Verification items for the finished model (mm, model axes). Give positions to 0.01 mm unless a question says otherwise; leave off trailing zeros. Order: outer loops, then holes, each group sorted by start corner. A loop starts at its lowest first (then second) coordinate and runs counter-clockwise, first axis right, second up. Notation, with made-up numbers: (27.25, 77) -> (70.25, 77) arc R12 ccw to (70.25, 96) -> close; hole circle Ø4 at (28.25, 73.5). An arc over 180 degrees is marked (long way). Return JSON: item names as keys, results as strings. Group by question number.
(1) Cross-section at B-B on x = 0. Enter the section's corners in (y, z).
(2) Cross-section at C-C on z = -23. Enter the section's corners in (x, y).
(3) Cross-section at D-D on x = -7. Enter the section's corners in (y, z), then the cut area to 3 significant figures.
(4) Thickness scan on line 1 along Z through (x, y) = (0, 1.25); line 2 along Z through (x, y) = (-23.5, 0.3); line 3 along X through (y, z) = (1.5, -5.5). Record the ranges inside material, lowest first.
(5) Depth check by flat-ended pin: pin 1 Ø5.5 at (x, z) = (0, 0) entering from -Y. Enter the tip coordinate at first touch or a pass-through.
(6) Cross-section at A-A on y = 1.2. Enter the section's corners in (x, z), then the cut area to 3 significant figures.
Autodesk Inventor part; units mm, degrees
ref_plane "YZ Plane" through (0, 0, 0) normal (1, 0, 0) x (0, 1, 0)
ref_plane "XZ Plane" through (0, 0, 0) normal (0, 1, 0) x (-1, 0, 0)
ref_plane "XY Plane" through (0, 0, 0) normal (0, 0, 1) x (1, 0, 0)
sketch "main" plane through (0, 0, 0) normal (0, 0, 1) x (1, 0, 0)
  circle A0 centre (31.4944, -42.9627) radius 2.1844
  arc A1 (31.4944, -49.3127) -> (37.7453, -41.8453) centre (31.4944, -42.9627) ccw
  arc A2 (-34.2347, -37.0168) -> (-32.0056, -49.3127) centre (-32.0056, -42.9627) ccw
  arc A3 (-34.2347, -37.0168) -> (27.8848, -9.8628) centre (-257.1487, 557.5708) ccw
  line L0 (37.7453, -41.8453) -> (32.4355, -12.1413)
  line L1 (-32.0056, -49.3127) -> (31.4944, -49.3127)
  arc A4 (32.4355, -12.1413) -> (27.8848, -9.8628) centre (29.31, -12.7) ccw
  circle A5 centre (-32.0056, -42.9627) radius 2.0955
  point P0 (5.1717, -33.3366)
  point P1 (31.6842, -7.9384)
  dimension "d0" = 1270
  dimension "d1" = 12.7
  dimension "d2" = 12.7
  dimension "d3" = 3.175
  dimension "d4" = 4.191
sketch "Sketch1" plane through (0, 0, 0) normal (0, 1, 0) x (-1, 0, 0)
  circle A0 centre (-0.1035, -63.4999) radius 2.1844
  arc A1 (-6.4535, -63.4896) -> (1.0037, -69.7526) centre (-0.1035, -63.4999) ccw
  arc A2 (5.9495, 2.2194) -> (-6.35, 0.0103) centre (0, 0) ccw
  arc A3 (5.9495, 2.2194) -> (33.0022, -59.9443) centre (600.8995, 224.1642) ccw
  line L0 (1.0037, -69.7526) -> (30.7163, -64.4912)
  line L1 (-6.35, 0.0103) -> (-6.4535, -63.4896)
  arc A4 (30.7163, -64.4912) -> (33.0022, -59.9443) centre (30.1627, -61.3648) ccw
  circle A5 centre (0, 0) radius 2.0955
  point P0 (0, 0)
extrude "Extrusion1" add sketch "Sketch1" along normal blind 1.5875
properties part number "Magazine Gusset" material "Acetal Resin, White"
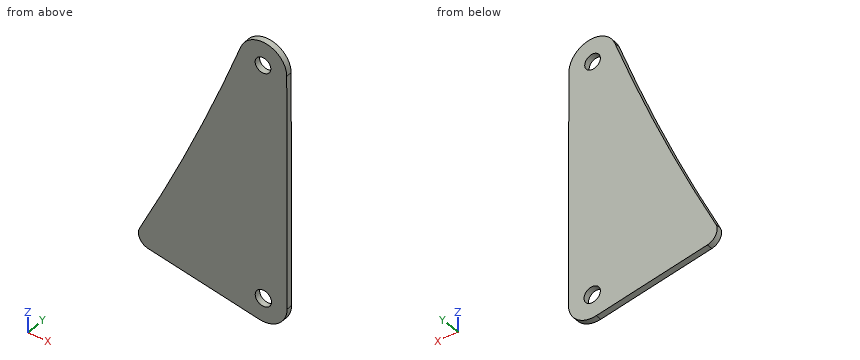
Verdict:
{
 "1": {"outline": "(0, -69.85) -> (1.59, -69.85) -> (1.59, -65.68) -> (0, -65.68) -> close; (0, -61.32) -> (1.59, -61.32) -> (1.59, -2.1) -> (0, -2.1) -> close; (0, 2.1) -> (1.59, 2.1) -> (1.59, 6.35) -> (0, 6.35) -> close"},
 "2": {"outline": "(-15.98, 0) -> (6.39, 0) -> (6.39, 1.59) -> (-15.98, 1.59) -> close"},
 "3": {"outline": "(0, -68.69) -> (1.59, -68.69) -> (1.59, -0.58) -> (0, -0.58) -> close", "area": "108 mm²"},
 "4": {"line 1": "-69.85 to -65.68, -61.32 to -2.1, 2.1 to 6.35", "line 2": "-65.77 to -40.1", "line 3": "-8.89 to 6.36"},
 "5": {"pin 1": "y = 0"},
 "6": {"outline": "(-33, -59.94) arc R3.17 ccw to (-30.72, -64.49) -> (-1, -69.75) arc R6.35 ccw to (6.45, -63.49) -> (6.35, 0.01) arc R6.35 ccw to (-5.95, 2.22) arc R635 cw to start; hole circle Ø4.19 at (0, 0); hole circle Ø4.37 at (0.1, -63.5)", "area": "1,860 mm²"}
}
